Input: part model. Units: mm. Frame: model coordinates. Give positions to 0.01 mm unless a question says otherwise; leave off trailing zeros. Write each loop counter-clockwise with the first axis right and the second up, starting at its lowest first coordinate (ties: lowest second). Pieces come first, ordered by that corner, then holes.
```python
from build123d import *

# Parameters (mm, degrees)
SKETCH1_R           = 9.2075
BOSS_EXTRUDE1_DEPTH = 9.25
BOSS_EXTRUDE1_TAPER = 2
SKETCH2_R           = 2.54
CUT_EXTRUDE1_DEPTH  = 23.623132407
FILLET1_R           = 1


with BuildPart() as part:
    # Sketch1 → Boss-Extrude1 (new body)
    with BuildSketch(Plane(origin=(0, 0, 0), x_dir=(1, 0, 0), z_dir=(0, 1, 0))):
        Circle(SKETCH1_R)
    boss_extrude1 = extrude(amount=BOSS_EXTRUDE1_DEPTH, taper=BOSS_EXTRUDE1_TAPER)

    # Mirror1: Boss-Extrude1 across plane
    add(boss_extrude1.mirror(Plane.ZX))

    # Sketch2 → Cut-Extrude1 (cut, through all)
    with BuildSketch(Plane(origin=(0, -9.25, 0), x_dir=(-1, 0, 0), z_dir=(0, -1, 0))):
        with Locations(Location((0, 0, 0), (0, 0, 90))):
            Circle(SKETCH2_R)
    extrude(amount=-CUT_EXTRUDE1_DEPTH, mode=Mode.SUBTRACT)

    # Fillet1
    fillet1_edges = [part.edges().sort_by_distance(p)[0] for p in [
        (-8.884482882, 9.25, 0),
        (-8.884482882, -9.25, 0),
    ]]
    fillet(fillet1_edges, radius=FILLET1_R)


solid = part.part
```
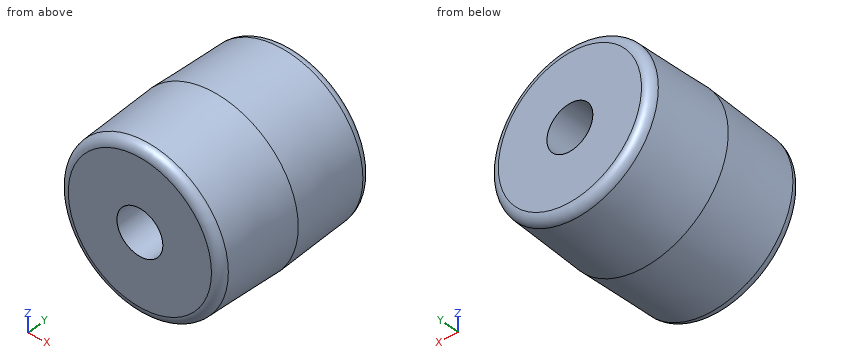
Item 1: Pin query (flat end, axial travel): pin 1 (2 mm diameter, centred on y = -7, z = -2.5, fed in from -X); pin 2 (3 mm diameter, centred on x = 2, y = 5.5, fed in from +Z); pin 3 (3 mm diameter, centred on x = -5, y = -2.5, fed in from -Z). Return the tip coordinate at first contact, or that it passes through.
Item 2: Section B-B (y = 3.5). Return loops of the section in (x, z).
Item 3: Ray query, line 1 (Z direction, x = 0.25, y = 6.25); line 2 (Z direction, x = 0.5, y = -8.25); line 3 (X direction, y = -0.75, z = -2). Return the intervals inside material, ascending.
Item 4: Section C-C (y = -4.25). Return loops of the section in (x, z).
Item 5: Section A-A (x = 0). Return loops of the section in (y, z), and give its area (3 significant figures).
Solved:
1. pin 1: stops at x = -8.84
1. pin 2: stops at z = 9.01
1. pin 3: stops at z = -8.42
2. outline: circle Ø18.17 at (0, 0); hole circle Ø5.08 at (0, 0)
3. line 1: z = -8.99 to -2.53, 2.53 to 8.99
3. line 2: z = -8.91 to -2.49, 2.49 to 8.91
3. line 3: x = -8.96 to -1.57, 1.57 to 8.96
4. outline: circle Ø18.12 at (0, 0); hole circle Ø5.08 at (0, 0)
5. outline: (-9.25, -7.92) arc R1 ccw to (-8.28, -8.92) - (0, -9.21) - (8.28, -8.92) arc R1 ccw to (9.25, -7.92) - (9.25, -2.54) - (-9.25, -2.54) - close; (-9.25, 2.54) - (9.25, 2.54) - (9.25, 7.92) arc R1 ccw to (8.28, 8.92) - (0, 9.21) - (-8.28, 8.92) arc R1 ccw to (-9.25, 7.92) - close
5. area: 240 mm2
